Verification items for the finished model (mm, model axes). A direction names the side the tool comes from. Round coordinates to 2 decimals unless told otherwise and drop trailing zeros. Loops run counter-clockwise (first coordinate to the right, second up) from the corner with the lowest first, then second, coordinate; pieces in that order, holes last. Notation, with made-up numbers: (-32.75, -12) -> (-5.75, -12) arc R22 ccw to (-5.75, -4) -> close; hole circle Ø2 at (33.25, 50.5). An arc over 180 degrees is marked (long way). Write item = value, one per line.
```python
from build123d import *

# Parameters (mm, degrees)
BOSS_EXTRUDE1_DEPTH                       = 15.9004
SKETCH2_R                                 = 15.9004
CUT_EXTRUDE1_DEPTH                        = 2.54
CUT_EXTRUDE1_DEPTH_BACK                   = 18.796
CBORE_FOR_5_16_HEX_HEAD_BOLT1_D           = 8.4328
CBORE_FOR_5_16_HEX_HEAD_BOLT1_CBORE_D     = 20.6375
CBORE_FOR_5_16_HEX_HEAD_BOLT1_CBORE_DEPTH = 5.969
F_5_16_18_TAPPED_HOLE1_D                  = 6.5278
CUT_EXTRUDE2_DEPTH                        = 40.894


with BuildPart() as part:
    # Sketch1 → Boss-Extrude1 (new body)
    with BuildSketch(Plane.XY):
        with BuildLine():
            Line((50.8, -20.32), (-50.8, -20.32))
            ThreePointArc((-50.8, -20.32), (-71.12, 0), (-50.8, 20.32))
            Line((-50.8, 20.32), (50.8, 20.32))
            Line((50.8, 20.32), (50.8, -20.32))
        make_face()
    extrude(amount=BOSS_EXTRUDE1_DEPTH)

    # Sketch2 → Cut-Extrude1 (cut, two sides)
    with BuildSketch(Plane(origin=(2.48157472, 0, 15.9004), x_dir=(1, 0, 0), z_dir=(0, 0, 1))) as cut_extrude1_sk:
        with Locations((-53.28157472, 0)):
            Circle(SKETCH2_R)
    extrude(amount=CUT_EXTRUDE1_DEPTH, mode=Mode.SUBTRACT)
    extrude(cut_extrude1_sk.sketch, amount=-CUT_EXTRUDE1_DEPTH_BACK, mode=Mode.SUBTRACT)

    # CBORE for 5/16 Hex Head Bolt1 (through all)
    with Locations(Plane(origin=(0, 0, 0), x_dir=(-1, 0, 0), z_dir=(0, 0, -1))):
        with Locations((-36.83, 0), (1.27, 0)):
            CounterBoreHole(CBORE_FOR_5_16_HEX_HEAD_BOLT1_D / 2, CBORE_FOR_5_16_HEX_HEAD_BOLT1_CBORE_D / 2, CBORE_FOR_5_16_HEX_HEAD_BOLT1_CBORE_DEPTH)

    # 5/16-18 Tapped Hole1 (through all)
    with Locations(Plane(origin=(0, -20.32, 0), x_dir=(-1, 0, 0), z_dir=(0, -1, 0))):
        with Locations((50.8, -7.9502)):
            Hole(F_5_16_18_TAPPED_HOLE1_D / 2)

    # Sketch10 → Cut-Extrude2 (cut)
    with BuildSketch(Plane.XZ.offset(20.32)):
        with BuildLine():
            Line((-50.8, 15.9004), (-71.468119006, 15.9004))
            Line((-71.468119006, 15.9004), (-71.468119006, 0))
            Line((-71.468119006, 0), (-50.8, 0))
            ThreePointArc((-50.8, 0), (-58.7502, 7.9502), (-50.8, 15.9004))
        make_face()
    extrude(amount=-CUT_EXTRUDE2_DEPTH, mode=Mode.SUBTRACT)


solid = part.part
```
(1) Material ranges on probe 1 along X at (y, z) = (-9.5, 4); probe 2 along Y at (x, z) = (-1.27, 9); probe 3 along X at (y, z) = (-0.5, 11.25), recorded low to high. Write a range as from..to.
Filled sheet:
probe_1 = -38.05..-5.3, 2.76..32.8, 40.86..50.8
probe_2 = -20.32..-4.22, 4.22..20.32
probe_3 = -34.91..-5.46, 2.92..32.64, 41.02..50.8
(2) Set-up check for faces 1 (the face through (0.967, -10.073, 2.943)), 2 (the face through (12, 0, 0)): record each of +Z, -Z, +X, -X, +Y, -Y from which the full face is reachable in a straight line by a thin tool's end or side.
Filled sheet:
face_1 = -Z
face_2 = -Z, +X, -X, +Y, -Y
(3) Sectioned sample at D-D, the plane z = 3.25. Record the cut outline in (x, y), and give its area (3 significant figures).
Filled sheet:
outline = (-57.21, -19.28) arc R20.32 ccw to (-50.8, -20.32) -> (50.8, -20.32) -> (50.8, 20.32) -> (-50.8, 20.32) arc R20.32 ccw to (-57.21, 19.28) -> (-57.21, 14.55) arc R15.9 cw (long way) to (-57.21, -14.55) -> close; hole circle Ø20.64 at (-1.27, 0); hole circle Ø20.64 at (36.83, 0)
area = 3,120 mm2
(4) Sectioned sample at C-C, the plane y = -2. Record the cut outline in (x, z), and give its area (3 significant figures).
Filled sheet:
outline = (-35.03, 0) -> (-11.39, 0) -> (-11.39, 5.97) -> (-4.98, 5.97) -> (-4.98, 15.9) -> (-35.03, 15.9) -> close; (2.44, 5.97) -> (8.85, 5.97) -> (8.85, 0) -> (26.71, 0) -> (26.71, 5.97) -> (33.12, 5.97) -> (33.12, 15.9) -> (2.44, 15.9) -> close; (40.54, 5.97) -> (46.95, 5.97) -> (46.95, 0) -> (50.8, 0) -> (50.8, 15.9) -> (40.54, 15.9) -> close
area = 976 mm2
(5) Sectioned sample at B-B, the plane z = 9.25. Record the cut outline in (x, y).
Filled sheet:
outline = (-58.64, -18.75) arc R20.32 ccw to (-53.79, -20.1) -> (-53.79, -15.62) arc R15.9 cw to (-58.64, -13.83) -> close; (-58.64, 13.83) arc R15.9 cw to (-53.79, 15.62) -> (-53.79, 20.1) arc R20.32 ccw to (-58.64, 18.75) -> close; (-47.81, -20.32) -> (50.8, -20.32) -> (50.8, 20.32) -> (-47.81, 20.32) -> (-47.81, 15.62) arc R15.9 cw to (-47.81, -15.62) -> close; hole circle Ø8.43 at (-1.27, 0); hole circle Ø8.43 at (36.83, 0)
(6) Draft check along Z on faces 3 (the face through (-47.687, 17.966, 6.97)), 4 (the face through (-58.75, -17.09, 7.78)), 5 (the face through (45, -6.3, 2.9)), 6 (the face through (-54.06, -17.9, 7.81)). Enter one of: released by +Z, released by -Z, zero draft, split by the parting line, or undercut.
Filled sheet:
face_3 = undercut
face_4 = split by the parting line
face_5 = zero draft
face_6 = undercut
(7) Go/stop test with a flat-tipped pin: pin 1 Ø7.5 at (x, y) = (-1.27, 0) entering from -Z. Record where the tip stops, or that it passes through.
Filled sheet:
pin_1 = through
(8) Sectioned sample at A-A, the plane x = 36.83. Record the cut outline in (y, z).
Filled sheet:
outline = (-20.32, 0) -> (-10.32, 0) -> (-10.32, 5.97) -> (-4.22, 5.97) -> (-4.22, 15.9) -> (-20.32, 15.9) -> close; (4.22, 5.97) -> (10.32, 5.97) -> (10.32, 0) -> (20.32, 0) -> (20.32, 15.9) -> (4.22, 15.9) -> close
